from build123d import *

# Parameters (mm, degrees)
BOSS_EXTRUDE1_DEPTH        = 3.175
F_1_4_CLEARANCE_HOLE2_D    = 6.7564
F_1_4_CLEARANCE_HOLE1_D    = 6.7564
FILLET1_R                  = 2.54
F_10_CLEARANCE_HOLE1_D     = 5.1054
F_10_CLEARANCE_HOLE1_DEPTH = 3.175


with BuildPart() as part:
    # Sketch1 → Boss-Extrude1 (new body)
    with BuildSketch(Plane(origin=(0, 0, 0), x_dir=(1, 0, 0), z_dir=(0, 1, 0))):
        with BuildLine():
            Line((0, 50.8), (19.05, 50.8))
            ThreePointArc((19.05, 50.8), (56.03836137, 31.046405743), (81.899154962, -1.962119182))
            ThreePointArc((81.899154962, -1.962119182), (79.082321477, -10.420655433), (70.584022136, -7.726162031))
            ThreePointArc((70.584022136, -7.726162031), (46.770595677, 9.16746016), (19.05, 0))
            Line((19.05, 0), (0, 0))
            Line((0, 0), (0, 50.8))
        make_face()
    extrude(amount=BOSS_EXTRUDE1_DEPTH)

    # 1/4 Clearance Hole2 (through all)
    with Locations(Plane(origin=(0, 0, 0), x_dir=(-1, 0, 0), z_dir=(0, -1, 0))):
        with Locations((-76.2, -4.7625)):
            Hole(F_1_4_CLEARANCE_HOLE2_D / 2)

    # 1/4 Clearance Hole1 (through all)
    with Locations(Plane(origin=(0, 3.175, 0), x_dir=(1, 0, 0), z_dir=(0, 1, 0))):
        with Locations((9.525, 36.5125), (9.525, 14.2875)):
            Hole(F_1_4_CLEARANCE_HOLE1_D / 2)

    # Fillet1
    fillet1_edges = [part.edges().sort_by_distance(p)[0] for p in [
        (0, 1.5875, -50.8),
        (19.05, 1.5875, -50.8),
        (19.05, 1.5875, 0),
        (0, 1.5875, 0),
    ]]
    fillet(fillet1_edges, radius=FILLET1_R)

    # #10 Clearance Hole1
    with Locations(Plane(origin=(0, 3.175, 0), x_dir=(1, 0, 0), z_dir=(0, 1, 0))):
        with Locations((41.275, 25.437101907)):
            Hole(F_10_CLEARANCE_HOLE1_D / 2, depth=F_10_CLEARANCE_HOLE1_DEPTH)


solid = part.part
Build history of the part. All positions in model axes, mm. A direction names the side the tool comes from. Coordinates: 2 decimals unless noted, no trailing zeros. Write each loop counter-clockwise with the first axis right and the second up, starting at its lowest first coordinate (ties: lowest second). Pieces come first, ordered by that corner, then holes.
(1) Cut at A-A on z = -6. List the corners of the cut face in (x, y) (3 decimals).
(2) Cut at B-B on x = 76.2. List the corners of the cut face in (y, z) (1 decimal).
(3) Cut at D-D on z = -18.5. List the corners of the cut face in (x, y) (1 decimal), and give its area (3 significant figures).
(4) 3-axis set-ups, long thin cutter, end or side, ignore diameter. For faces 5 (the cylindrical face through (18.944, 1.61, -0.175)), 6 (the flat face through (33, 3.175, -20)), 7 (the flat face through (10, 2, 0)): which of +Z, -Z, +X, -X, +Y, -Y reach the whole face in a straight line?
(5) Mould opens along X. For faces 1 (the cylindrical face through (7.97, 1.57, -11.29)), 2 (the cylindrical face through (40.1, 1.57, -23.17)), 3 (the cylindrical face through (0.724, 1.61, -0.764)), 4 (the flat face through (33, 0, -20)) say: pulls with the +X half, pulls with the -X half, needs draft (parallel to the pull), parting line crosses it, or undercut.
(6) Cut at C-C on y = 0.9. State how many separate pieces and enclosed holes the cut face has, and give its area (3 significant figures).
(7) Drill centre lines: line 1 (Z direction, x = 15, y = 0.35); line 2 (X direction, y = 2.05, z = 3); line 3 (X direction, y = 0.25, z = -2). Where is each one in solid material? Low to high.
(8) Pin check, flat tip, straight feed: pin 1 Ø1 at (x, y) = (11.5, 1) entering from +Z. Stop position of the tip, or through.
Working result:
1. outline: (0, 0) - (27.29, 0) - (27.29, 3.175) - (0, 3.175) - close; (56.659, 0) - (77.535, 0) - (77.535, 3.175) - (56.659, 3.175) - close
2. outline: (0, -8.1) - (3.2, -8.1) - (3.2, 1.4) - (0, 1.4) - close; (0, 8.1) - (3.2, 8.1) - (3.2, 11.1) - (0, 11.1) - close
3. outline: (0, 0) - (68.6, 0) - (68.6, 3.2) - (0, 3.2) - close
3. area: 218 mm2
4. face 5: +Z, +Y, -Y
4. face 6: +Z, -Z, +X, -X, +Y
4. face 7: +Z, -X, +Y, -Y
5. face 1: undercut
5. face 2: undercut
5. face 3: pulls with the -X half
5. face 4: needs draft
6. separate pieces: 1
6. enclosed holes: 4
6. area: 2,680 mm2
7. line 1: z = -50.8 to 0
7. line 2: x = 67.54 to 73.32, 79.08 to 82.3
7. line 3: x = 0.06 to 21.23, 62.72 to 79.84
8. pin 1: stops at z = 0
